Part model, mm, in its own coordinate system. A direction names the side the tool comes from. Give positions to 0.01 mm unless a question says otherwise; leave off trailing zeros. Loops run counter-clockwise (first coordinate to the right, second up) from the corner with the lowest first, then second, coordinate; pieces in that order, holes last. Notation, with made-up numbers: M -10,-19 L 14,-19 A28 ccw 14,7 Z; hole C 21.5,33 d8. An arc over 180 degrees is marked long. Put each result on its own line as item: value. Start each with the question number.
```python
from build123d import *

# Parameters (mm, degrees)
BOX173_W               = 0.8
BOX173_H               = 16
BOX173_DEPTH           = 0.8
BOX174_W               = 0.8
BOX174_H               = 16
BOX174_DEPTH           = 0.8
CUT090_PLACEMENT_ANGLE = 189


with BuildPart() as cubo173:
    # Box173 → Box173 (new body)
    with BuildSketch(Plane.XY):
        with Locations((0.4, 8)):
            Rectangle(BOX173_W, BOX173_H)
    extrude(amount=BOX173_DEPTH)


with BuildPart() as obj1:
    # Box174 → Box174 (new body)
    with BuildSketch(Plane(origin=(0.3, 0, 0.3), x_dir=(1, 0, 0), z_dir=(0, 0, 1))):
        with Locations((0.4, 8)):
            Rectangle(BOX174_W, BOX174_H)
    extrude(amount=BOX174_DEPTH)

    # Cut090: cut Cubo173
    add(cubo173.part, mode=Mode.SUBTRACT)


with BuildPart() as obj1_1:
    # Cut090 placement: moved
    add(obj1.part.moved(Location((-170.3, 159.8, -1.45))).rotate(Axis((-170.3, 159.8, -1.45), (0, 0, 1)), CUT090_PLACEMENT_ANGLE))


solid = obj1_1.part
```
1) Wall check: L1, parallel to X at y = 153, z = -0.8; L2, parallel to X at y = 154.5, z = -0.45. Give the ranges that are in metal, low to high.
2) Band-saw the part on A-A on x = -170.85. Give the cut face in (y, z).
3) Band-saw the part on B-B on y = 153.5. Give the cut face in (x, z).
4) Which spindle directions (+Z, -Z, +X, -X, +Y, -Y) get a long thin tool onto all of the face, cutting with end or side? Do faces 1 (the flat face through (-169.36, 151.96, -0.5)), 2 (the flat face through (-169.856, 151.884, -0.904)). Say none if no direction does.
5) Band-saw the part on C-C on z = -1. Give the cut face in (x, y).
6) Pin check, flat tip, straight feed: pin 1 Ø1.5 at (x, y) = (-169, 153.5) entering from -Z. Stop position of the tip, or through.
Evaluation:
1. L1: -170.34 to -170.03
1. L2: -170.57 to -169.76
2. outline: M 156.24,-1.15 L 158.16,-1.15 L 158.16,-0.65 L 159.71,-0.65 L 159.71,-0.35 L 156.24,-0.35 Z
3. outline: M -170.42,-1.15 L -170.11,-1.15 L -170.11,-0.65 L -169.61,-0.65 L -169.61,-0.35 L -170.42,-0.35 Z
4. face 1: +Z, -Z, +X, +Y
4. face 2: -Z, +X, +Y
5. outline: M -171.39,159.63 L -168.88,143.82 L -168.59,143.87 L -171.09,159.67 Z
6. pin 1: z = -0.65
